from build123d import *

# Parameters (mm, degrees)
F1_DEPTH = 8.5
F3_D     = 8
F3_DEPTH = 0.5
F3_TIP   = 2.4034424761
F4_D     = 4
F4_DEPTH = 12
F4_START = 1.7017212
F4_TIP   = 1.2017212381


with BuildPart() as f1:
    # F0 (on Top) → F1 (new body)
    with BuildSketch(Plane.XY):
        with BuildLine():
            ThreePointArc((-8.8450443894, 11.325138621), (7.7049556106, 17.425138621), (24.2549556106, 11.325138621))
            Line((24.2549556106, 11.325138621), (39.2549556106, 11.325138621))
            Line((39.2549556106, 11.325138621), (39.2549556106, 16.325138621))
            Line((39.2549556106, 16.325138621), (24.2549556106, 16.325138621))
            ThreePointArc((24.2549556106, 16.325138621), (7.7049556106, 22.425138621), (-8.8450443894, 16.325138621))
            Line((-8.8450443894, 16.325138621), (-23.8450443894, 16.325138621))
            Line((-23.8450443894, 16.325138621), (-23.8450443894, 11.325138621))
            Line((-23.8450443894, 11.325138621), (-8.8450443894, 11.325138621))
        make_face()
    extrude(amount=F1_DEPTH)

    # F3
    with Locations(Plane(origin=(0, 16.325138621, 0), x_dir=(-1, 0, 0), z_dir=(0, 1, 0))):
        with Locations((-31.7569042742, 4.25), (16.3450443894, 4.25)):
            Hole(F3_D / 2, depth=F3_DEPTH)
            with Locations((0, 0, -(F3_DEPTH + F3_TIP / 2))):  # 118° drill point
                Cone(0, F3_D / 2, F3_TIP, mode=Mode.SUBTRACT)

    # F4
    # its depths count from where the whole tool has entered the part; down to there all is cleared
    with Locations(Plane(origin=(0, 16.325138621, 0), x_dir=(-1, 0, 0), z_dir=(0, 1, 0)).offset(-F4_START)):
        with Locations((-31.7569042742, 4.25), (16.3450443894, 4.25)):
            Hole(F4_D / 2, depth=F4_DEPTH)
            with Locations((0, 0, -(F4_DEPTH + F4_TIP / 2))):  # 118° drill point
                Cone(0, F4_D / 2, F4_TIP, mode=Mode.SUBTRACT)


solid = f1.part
Design review of the part built by this model. Coordinates are the model's own, in mm. A direction names the side the tool comes from. Give positions to 0.01 mm unless a question says otherwise; leave off trailing zeros. Order: outer loops, then holes, each group sorted by start corner. A loop starts at its lowest first (then second) coordinate and runs counter-clockwise, first axis right, second up. Notation, with made-up numbers: (0, -23) - (23, -23) arc R32 ccw to (23, 7) - close; hole circle Ø8 at (-3, 74.25). An arc over 180 degrees is marked (long way). Use CSV: the item, a comma, the result in double quotes. Start each with the question number.
Q1. Take a section at B-B (x = -11). State the section outline as (y, z) points, and give its area (3 significant figures).
Q2. Take a section at A-A (z = 4.25). State the section outline as (x, y) points, and give its area (3 significant figures).
Q3. Draft analysis for pull direction X (two halves, no side actions). For faces 6 (the face through (7, 18, 8.5)), 7 (the face through (39.255, 14, 4)), 8 (the face through (-12.65, 16.07, 2.72)), 9 (the face through (-23.845, 14, 4)), state which applies: pulls with the +X half, pulls with the -X half, needs draft (parallel to the pull), parting line crosses it, or undercut.
Q4. For P1, Ø2, axis at y = 21, z = 3, coming from the -X side; P2, Ø2, axis at x = -11, z = 2.5, coming from the +Y side; P3, Ø1.5, axis at y = 17.5, z = 4.5, coming from the +X side; P4, Ø3.5, axis at x = 31.76, z = 4.25, coming from the -Y side, all flat-tipped, find the tip position at first contact; note any pin that passes through.
Q5. Take a section at C-C (y = 18.5). State the section outline as (x, z) points, and give its area (3 significant figures).
Q6. For line 1 (X direction, y = 12.8, z = 4.25); line 2 (X direction, y = 13.35, z = 4.25); line 3 (Y direction, x = 36.5, z = 4.25), list the stretches that pass through material, from the lowest coordinate up.
Q7. Machinability: for faces 1 (the face through (7, 18, 0)), 2 (the face through (35.452, 16.072, 2.718)), 3 (the face through (7.453, 17.424, 4.19)), 4 (the face through (34, 16.325, 8)), 5 (the face through (-14.6, 16.325, 0.4)), which of the approach directions +Z, -Z, +X, -X, +Y, -Y give a long, thin tool a straight path to every point of the face, cutting with its end or side? Answer none if there is none.
Calculated:
1,outline,"(11.33, 0) - (16.33, 0) - (16.33, 8.5) - (11.33, 8.5) - close"
1,area,"42.5 mm²"
2,outline,"(-23.85, 11.33) - (-18.35, 11.33) - (-18.35, 14.62) - (-20.35, 15.83) - (-20.35, 16.33) - (-23.85, 16.33) - close; (-14.35, 11.33) - (-8.85, 11.33) arc R25.5 cw to (24.25, 11.33) - (29.76, 11.33) - (29.76, 14.62) - (27.76, 15.83) - (27.76, 16.33) - (24.25, 16.33) arc R25.5 ccw to (-8.85, 16.33) - (-12.35, 16.33) - (-12.35, 15.83) - (-14.35, 14.62) - close; (33.76, 11.33) - (39.25, 11.33) - (39.25, 16.33) - (35.76, 16.33) - (35.76, 15.83) - (33.76, 14.62) - close"
2,area,"267 mm²"
3,face 6,"needs draft"
3,face 7,"pulls with the +X half"
3,face 8,"undercut"
3,face 9,"pulls with the -X half"
4,P1,"stops at x = -3.15"
4,P2,"stops at y = 16.33"
4,P3,"stops at x = 23.74"
4,P4,"passes through"
5,outline,"(-5.89, 0) - (21.3, 0) - (21.3, 8.5) - (-5.89, 8.5) - close"
5,area,"231 mm²"
6,line 1,"x = -23.85 to -18.35, -14.35 to -6.94, 22.35 to 29.76, 33.76 to 39.25"
6,line 2,"x = -23.85 to -18.35, -14.35 to -6.12, 21.53 to 29.76, 33.76 to 39.25"
6,line 3,"y = 11.33 to 16.33"
7,face 1,"-Z, +X, -X, +Y, -Y"
7,face 2,"+Y"
7,face 3,"+Z, -Z, -Y"
7,face 4,"+Z, -Z, +X, +Y"
7,face 5,"+Z, -Z, -X, +Y"
